```python
from build123d import *

# Parameters (mm, degrees)
CUT_EXTRUDE2_REACH = 237.261
MOTOR_HOLE_R       = 18.415
SKETCH1_R          = 3.25
CUT_EXTRUDE3_DEPTH = 236.261075795
FILLET2_R          = 25.4


with BuildPart() as part:
    # Compartment → Revolve1 (revolve)
    with BuildSketch(Plane.XY, mode=Mode.PRIVATE) as revolve1_sk:
        Polygon((120.65, -80), (0, -80), (0, -75), (118.11, -75), (118.11, 81.972), (120.65, 81.972), align=None)
    revolve(revolve1_sk.sketch.rotate(Axis((0, 0, 0), (0, 1, 0)), 90), axis=Axis((0, 0, 0), (0, 1, 0)))

    # Motor Hole → Cut-Extrude2 (cut, up to next)
    with BuildSketch(Plane.XZ.offset(80), mode=Mode.PRIVATE) as cut_extrude2_sk1:
        with Locations(Location((0, 0, 0), (0, 0, 270))):
            Circle(MOTOR_HOLE_R)
    cut_extrude2_tool1 = extrude(cut_extrude2_sk1.sketch, amount=-CUT_EXTRUDE2_REACH, mode=Mode.PRIVATE) & part.part
    add(cut_extrude2_tool1.solids().sort_by_distance((0, -80, 0))[0], mode=Mode.SUBTRACT)

    # Sketch1 → Cut-Extrude3 (cut, through all)
    with BuildSketch(Plane.XZ.offset(80)):
        with Locations(Location((0, 63.5, 0), (0, 0, 270))):
            Circle(SKETCH1_R)
        with Locations(Location((0, -63.5, 0), (0, 0, 270))):
            Circle(SKETCH1_R)
        with Locations(Location((63.5, 0, 0), (0, 0, 270))):
            Circle(SKETCH1_R)
        with Locations(Location((-63.5, 0, 0), (0, 0, 270))):
            Circle(SKETCH1_R)
    extrude(amount=-CUT_EXTRUDE3_DEPTH, mode=Mode.SUBTRACT)

    # Fillet2
    fillet2_edges = [part.edges().sort_by_distance(p)[0] for p in [
        (0, -75, 118.11),
        (0, -80, 120.65),
    ]]
    fillet(fillet2_edges, radius=FILLET2_R)


solid = part.part
```
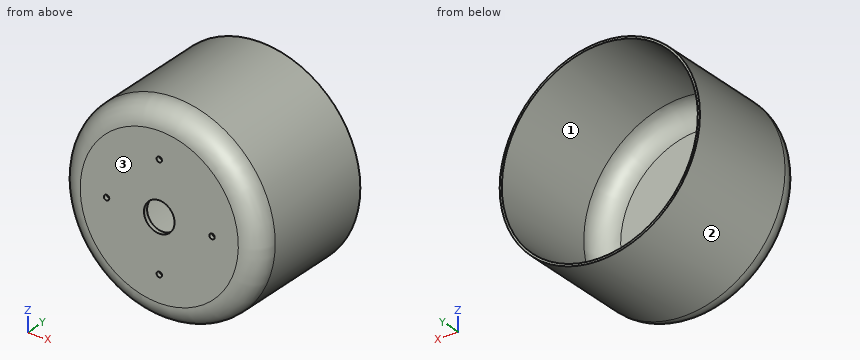
Geometry check sheet. Reference: the model listing, model coordinates, mm. Face numbers are marked on the shaded views. Round coordinates to 2 decimals unless told otherwise and drop trailing zeros. Write each loop counter-clockwise with the first axis right and the second up, starting at its lowest first coordinate (ties: lowest second). Pieces come first, ordered by that corner, then holes. Notation, with made-up numbers: (46.25, 82.25) - (58.25, 82.25) arc R34 ccw to (58.25, 115.25) - close; hole circle Ø11 at (-30.5, 31). An arc over 180 degrees is marked (long way). Write each question's results on one line, items separated by ' | '.
(1) Sectioned sample at C-C, the plane y = -42.5. Enter the section's corners in (x, z), plus the area to 3 significant figures.
Computed:
outline: circle Ø241.3 at (0, 0); hole circle Ø236.22 at (0, 0) | area: 1,910 mm^2
(2) Draft check along Z on the marked faces 1, 2 and 3. Enter one of: pulls with the +Z half, pulls with the -Z half, needs draft (parallel to the pull), parting line crosses it, or undercut.
Computed:
face 1: undercut | face 2: parting line crosses it | face 3: needs draft
(3) Sectioned sample at A-A, the plane x = 0. Enter the section's corners in (y, z) (3 decimals), plus the area to 3 significant figures.
Computed:
outline: (-80, -95.25) arc R25.4 ccw to (-54.6, -120.65) - (81.972, -120.65) - (81.972, -118.11) - (-49.6, -118.11) arc R25.4 cw to (-75, -92.71) - (-75, -66.75) - (-80, -66.75) - close; (-80, -60.25) - (-75, -60.25) - (-75, -18.415) - (-80, -18.415) - close; (-80, 18.415) - (-75, 18.415) - (-75, 60.25) - (-80, 60.25) - close; (-80, 66.75) - (-75, 66.75) - (-75, 92.71) arc R25.4 cw to (-49.6, 118.11) - (81.972, 118.11) - (81.972, 120.65) - (-54.6, 120.65) arc R25.4 ccw to (-80, 95.25) - close | area: 1,750 mm^2
(4) Sectioned sample at B-B, the plane z = 0. Enter the section's corners in (x, y) (3 decimals), plus the area to 3 significant figures.
Computed:
outline: (-120.65, -54.6) arc R25.4 ccw to (-95.25, -80) - (-66.75, -80) - (-66.75, -75) - (-92.71, -75) arc R25.4 cw to (-118.11, -49.6) - (-118.11, 81.972) - (-120.65, 81.972) - close; (-60.25, -80) - (-18.415, -80) - (-18.415, -75) - (-60.25, -75) - close; (18.415, -80) - (60.25, -80) - (60.25, -75) - (18.415, -75) - close; (66.75, -80) - (95.25, -80) arc R25.4 ccw to (120.65, -54.6) - (120.65, 81.972) - (118.11, 81.972) - (118.11, -49.6) arc R25.4 cw to (92.71, -75) - (66.75, -75) - close | area: 1,750 mm^2
(5) Depth check by flat-ended pin: pin 1 Ø1.5 at (y, z) = (4, 21) entering from -X; pin 2 Ø1 at (x, z) = (40, 12.5) entering from +Y; pin 3 Ø6 at (y, z) = (17, 36) entering from +X. Enter the tip coordinate at first touch or a pass-through.
Computed:
pin 1: stops at x = -118.94 | pin 2: stops at y = -75 | pin 3: stops at x = 116.05
(6) Thickness scan on probe 1 along X at (y, z) = (8, 0); probe 2 along X at (y, z) = (-76.5, 0) (3 decimals); probe 3 along Y at (x, z) = (-24, 76.5). Record the ranges inside material, lowest first. Write a range as from..to.
Computed:
probe 1: x = -120.65..-118.11, 118.11..120.65 | probe 2: x = -108.117..-66.75, -60.25..-18.415, 18.415..60.25, 66.75..108.117 | probe 3: y = -80..-75
